```python
from build123d import *

# Parameters (mm, degrees)
SKETCH2_W           = 203.2
SKETCH2_H           = 56.642
SKETCH2_R           = 2
SKETCH2_W_2         = 25.4
SKETCH2_H_2         = 13.97
BOSS_EXTRUDE1_DEPTH = 5.08
CUT_EXTRUDE1_DEPTH  = 4
BOSS_EXTRUDE2_START = -56.642
SKETCH5_W           = 6.35
SKETCH5_H           = 7.62
SKETCH5_R           = 1.5
SKETCH5_H_2         = 5.08
BOSS_EXTRUDE2_DEPTH = 3.81


with BuildPart() as part:
    # Sketch2 → Boss-Extrude1 (new body)
    with BuildSketch(Plane(origin=(0, 0, 0), x_dir=(1, 0, 0), z_dir=(0, 1, 0))):
        Rectangle(SKETCH2_W, SKETCH2_H)
        with Locations(Location((-19.05, 2.392044149, 0), (0, 0, 270))):
            Circle(SKETCH2_R, mode=Mode.SUBTRACT)
        with Locations((0, 15.727044149)):
            Rectangle(SKETCH2_W_2, SKETCH2_H_2, mode=Mode.SUBTRACT)
        with Locations(Location((19.05, 2.392044149, 0), (0, 0, 270))):
            Circle(SKETCH2_R, mode=Mode.SUBTRACT)
        with BuildLine():
            Line((51.503794476, 13.896514657), (51.503794476, 15.095394657))
            Line((51.503794476, 15.095394657), (53.703434476, 15.095394657))
            Line((53.703434476, 15.095394657), (53.703434476, 13.896514657))
            ThreePointArc((53.703434476, 13.896514657), (56.700855716, 12.057279355), (57.874114476, 8.742044149))
            ThreePointArc((57.874114476, 8.742044149), (49.28837927, 4.644802909), (51.503794476, 13.896514657))
        make_face(mode=Mode.SUBTRACT)
    extrude(amount=BOSS_EXTRUDE1_DEPTH)

    # Sketch4 → Cut-Extrude1 (cut)
    with BuildSketch(Plane.XZ):
        Polygon((-16.769466437, -6.342044149), (-14.488932873, -2.392044149), (-16.769466437, 1.557955851), (-21.330533563, 1.557955851), (-23.611067127, -2.392044149), (-21.330533563, -6.342044149), align=None)
        Polygon((16.769466437, -6.342044149), (14.488932873, -2.392044149), (16.769466437, 1.557955851), (21.330533563, 1.557955851), (23.611067127, -2.392044149), (21.330533563, -6.342044149), align=None)
    extrude(amount=-CUT_EXTRUDE1_DEPTH, mode=Mode.SUBTRACT)

    # Sketch5 → Boss-Extrude2 (add)
    # profile 1 of 4: a face of its own
    with BuildSketch(Plane.XY.offset(28.321).offset(BOSS_EXTRUDE2_START)):
        with Locations((-63.5, -3.81)):
            Rectangle(SKETCH5_W, SKETCH5_H)
        with Locations(Location((-63.5, -3.81, 0), (0, 0, 180))):
            Circle(SKETCH5_R, mode=Mode.SUBTRACT)
    # profile 2 of 4: a face of its own
    with BuildSketch(Plane.XY.offset(28.321).offset(BOSS_EXTRUDE2_START)):
        with Locations((-63.5, 2.54)):
            Rectangle(SKETCH5_W, SKETCH5_H_2)
    # profile 3 of 4: a face of its own
    with BuildSketch(Plane.XY.offset(28.321).offset(BOSS_EXTRUDE2_START)):
        with Locations((63.5, 2.54)):
            Rectangle(SKETCH5_W, SKETCH5_H_2)
    # profile 4 of 4: a face of its own
    with BuildSketch(Plane.XY.offset(28.321).offset(BOSS_EXTRUDE2_START)):
        with Locations((63.5, -3.81)):
            Rectangle(SKETCH5_W, SKETCH5_H)
        with Locations(Location((63.5, -3.81, 0), (0, 0, 180))):
            Circle(SKETCH5_R, mode=Mode.SUBTRACT)
    extrude(amount=BOSS_EXTRUDE2_DEPTH)


solid = part.part
```
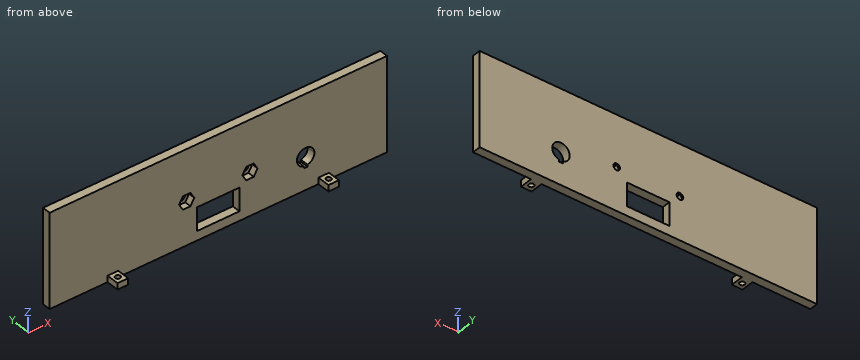
The listing builds one solid part. Answer for the finished solid, in the listing's coordinates (mm). Coordinates: 2 decimals unless noted, no trailing zeros. Write each loop counter-clockwise with the first axis right and the second up, starting at its lowest first coordinate (ties: lowest second). Pieces come first, ordered by that corner, then holes.
Q1. Given P1, Ø12, axis at x = 66.5, z = 5, coming from the -Y side; P2, Ø2.5, axis at x = 19.05, z = -2.39, coming from the -Y side, each flat-ended and moving along its own axis, determine where each tip first touches the part or whether it passes through.
Returned:
P1: stops at y = 0
P2: passes through
Q2. Section A-A, the plane x = 19.05 is taken. Write down the section's boundary in (y, z).
Returned:
outline: (0, -28.32) - (5.08, -28.32) - (5.08, -4.39) - (4, -4.39) - (4, -6.34) - (0, -6.34) - close; (0, 1.56) - (4, 1.56) - (4, -0.39) - (5.08, -0.39) - (5.08, 28.32) - (0, 28.32) - close
Q3. Section B-B, the plane y = 1.75 is taken. Write down the section's boundary in (x, z), then the cut area to 3 significant figures.
Returned:
outline: (-101.6, -28.32) - (101.6, -28.32) - (101.6, 28.32) - (-101.6, 28.32) - close; hole (-23.61, -2.39) - (-21.33, -6.34) - (-16.77, -6.34) - (-14.49, -2.39) - (-16.77, 1.56) - (-21.33, 1.56) - close; hole (-12.7, -22.71) - (12.7, -22.71) - (12.7, -8.74) - (-12.7, -8.74) - close; hole (14.49, -2.39) - (16.77, -6.34) - (21.33, -6.34) - (23.61, -2.39) - (21.33, 1.56) - (16.77, 1.56) - close; hole (51.5, -15.1) - (53.7, -15.1) - (53.7, -13.9) arc R5.27 ccw (long way) to (51.5, -13.9) - close
area: 11,000 mm2
Q4. Section D-D, the plane z = 3.5 is taken. Write down the section's boundary in (x, y), then the cut area to 3 significant figures.
Returned:
outline: (-101.6, 0) - (101.6, 0) - (101.6, 5.08) - (-101.6, 5.08) - close
area: 1,030 mm2
Q5. Section C-C, the plane z = -11.5 is taken. Write down the section's boundary in (x, y).
Returned:
outline: (-101.6, 0) - (-12.7, 0) - (-12.7, 5.08) - (-101.6, 5.08) - close; (12.7, 0) - (48.11, 0) - (48.11, 5.08) - (12.7, 5.08) - close; (57.09, 0) - (101.6, 0) - (101.6, 5.08) - (57.09, 5.08) - close
Q6. Find the intervals of material crossed by line 1 along X through (y, z) = (-3.81, -26.5) (3 decimals); line 2 along Z through (x, y) = (-19.05, 4.4); line 3 along Z through (x, y) = (-8.5, 3.5), in increasing order.
Returned:
line 1: x = -66.675 to -65, -62 to -60.325, 60.325 to 62, 65 to 66.675
line 2: z = -28.32 to -4.39, -0.39 to 28.32
line 3: z = -28.32 to -22.71, -8.74 to 28.32
